Check sheet for the modelled part. Datum: model origin and axes. Units: mm. Coordinates: 2 decimals unless noted, no trailing zeros. Order: outer loops, then holes, each group sorted by start corner. A loop starts at its lowest first (then second) coordinate and runs counter-clockwise, first axis right, second up.
1. Cross-section at A-A (x = 0). Enter the section's corners in (y, z), then the cut area to 3 significant figures.
2. Thickness scan on line 1 (Z direction, x = 0, y = -5); line 2 (Z direction, x = 5.5, y = -5.25); line 3 (X direction, y = -0.5, z = -27). Record the ranges inside material, lowest first.
3. Draft check along X on faces 1 (the flat face through (0, 0, 12)), 2 (the cylindrical face through (-2.423, -3.506, 26.134)). Enter one of: released by +X, released by -X, zero draft, split by the parting line, or undercut.
4. Gauge pin test, flat ends, axial feed: pin 1 Ø1 at (x, y) = (0.5, -4.5) entering from -Z; pin 2 Ø1 at (y, z) = (-6, -38.5) entering from -X; pin 3 Ø4 at (x, y) = (-9, -1) entering from -Z; pin 4 Ø3 at (y, z) = (-6.5, -6.5) entering from +X. Record the tip position at first contact, or that the pin passes through.
5. Cross-section at C-C (y = -2). Enter the section's corners in (x, z), then the cut area to 3 significant figures.
6. Cross-section at B-B (x = 13). Enter the section's corners in (y, z), then the cut area to 3 significant figures.
```python
from build123d import *

# Parameters (mm, degrees)
F0_R         = 11.176
F1_DEPTH     = 7.112
F2_T4_ANGLE  = 116.1586222886
F2_S5_R      = 15.24
F2_T6_DEPTH  = 30
F2_S7_R      = 15.24
F2_T8_DEPTH  = 30
F2_T12_ANGLE = 116.1586222886
F2_S13_R     = 15.24
F2_T14_DEPTH = 30
F2_S15_R     = 15.24
F2_T16_DEPTH = 30
F3_R         = 5.08
F4_T4_ANGLE  = 101.759749901
F4_S5_R      = 15.24
F4_T6_DEPTH  = 23
F4_S7_R      = 15.24
F4_T8_DEPTH  = 23
F4_T12_ANGLE = 101.7597499017
F4_S13_R     = 15.24
F4_T14_DEPTH = 27
F4_S15_R     = 15.24
F4_T16_DEPTH = 27
F4_T20_ANGLE = 101.7597499014
F4_S21_R     = 15.24
F4_T22_DEPTH = 27
F4_S23_R     = 15.24
F4_T24_DEPTH = 27
F4_T28_ANGLE = 101.7597499014
F4_S29_R     = 15.24
F4_T30_DEPTH = 27
F4_S31_R     = 15.24
F4_T32_DEPTH = 27


# Not quite as in the source:
# - a fillet or chamfer that OpenCascade refuses, or shapes differently, is made with other operations: its cross-section is extruded or revolved along the edge and cut away or added


with BuildPart() as f1:
    # F0 (on Front) → F1 (new body)
    with BuildSketch(Plane.XZ):
        with BuildLine():
            ThreePointArc((10.3608125449, -11.1763662883), (13.9670394713, -6.0974919769), (15.24, 0))
            ThreePointArc((15.24, 0), (13.9670394713, 6.0974919769), (10.3608125449, 11.1763662883))
            ThreePointArc((10.3608125449, 11.1763662883), (0, 15.24), (-10.3608125449, 11.1763662883))
            ThreePointArc((-10.3608125449, 11.1763662883), (-15.24, 0), (-10.3608125449, -11.1763662883))
            ThreePointArc((-10.3608125449, -11.1763662883), (0, -15.24), (10.3608125449, -11.1763662883))
        make_face()
        Circle(F0_R, mode=Mode.SUBTRACT)
        with BuildLine():
            ThreePointArc((-10.3608125449, 11.1763662883), (0, 15.24), (10.3608125449, 11.1763662883))
            ThreePointArc((10.3608125449, 11.1763662883), (9.1357508424, 18.8221602784), (10.8748760535, 26.3676480303))
            ThreePointArc((10.8748760535, 26.3676480303), (0, 21.8044767177), (-10.8748760535, 26.3676480303))
            ThreePointArc((-10.8748760535, 26.3676480303), (-9.1357508424, 18.8221602784), (-10.3608125449, 11.1763662883))
        make_face()
        with BuildLine():
            ThreePointArc((10.8748760535, -26.3676480303), (9.1357508424, -18.8221602784), (10.3608125449, -11.1763662883))
            ThreePointArc((10.3608125449, -11.1763662883), (0, -15.24), (-10.3608125449, -11.1763662883))
            ThreePointArc((-10.3608125449, -11.1763662883), (-9.1357508424, -18.8221602784), (-10.8748760535, -26.3676480303))
            ThreePointArc((-10.8748760535, -26.3676480303), (0, -21.8044767177), (10.8748760535, -26.3676480303))
        make_face()
        with BuildLine():
            ThreePointArc((-10.8748760535, 26.3676480303), (0, 21.8044767177), (10.8748760535, 26.3676480303))
            ThreePointArc((10.8748760535, 26.3676480303), (14.1065713598, 31.2771337877), (15.24, 37.0444767177))
            ThreePointArc((15.24, 37.0444767177), (-5.76734293, 51.1510480775), (-10.8748760535, 26.3676480303))
        make_face()
        with Locations((0, 37.0444767177)):
            Circle(F0_R, mode=Mode.SUBTRACT)
        with BuildLine():
            ThreePointArc((15.24, -37.0444767177), (14.1065713598, -31.2771337877), (10.8748760535, -26.3676480303))
            ThreePointArc((10.8748760535, -26.3676480303), (0, -21.8044767177), (-10.8748760535, -26.3676480303))
            ThreePointArc((-10.8748760535, -26.3676480303), (-5.76734293, -51.1510480775), (15.24, -37.0444767177))
        make_face()
        with Locations((0, -37.0444767177)):
            Circle(F0_R, mode=Mode.SUBTRACT)
    extrude(amount=F1_DEPTH)

    # F2: fillet of radius 5.08 on 2 edges, made by hand


with BuildPart() as f2_tool2:
    # F2_s3 → F2_t4 (revolve)
    with BuildSketch(Plane(origin=(29.8644460088, 0, -17.2301380427), x_dir=(0, 1, 0), z_dir=(0.8661774261, 0, -0.4997365971))):
        with BuildLine():
            ThreePointArc((-5.08, -21.2648569422), (-1.4878975516, -22.7527544938), (0, -26.3448569422))
            Line((0, -26.3448569422), (0, -21.2648569422))
            Line((0, -21.2648569422), (-5.08, -21.2648569422))
        make_face()
    revolve(axis=Axis((29.340401561, 0, -18.1384474874), (0, 1, 0)), revolution_arc=F2_T4_ANGLE)

    # F2_s5 → F2_t6 (cut, symmetric)
    with BuildSketch(Plane.XZ.offset(2.5)):
        with Locations((0, -37.0444767177)):
            Circle(F2_S5_R)
    extrude(amount=F2_T6_DEPTH, both=True, mode=Mode.SUBTRACT)

    # F2_s7 → F2_t8 (cut, symmetric)
    with BuildSketch(Plane.XZ.offset(2.5)):
        Circle(F2_S7_R)
    extrude(amount=F2_T8_DEPTH, both=True, mode=Mode.SUBTRACT)


with BuildPart() as f1_1:
    add(f1.part)

    # F2_t1: cut F2_tool2
    add(f2_tool2.part, mode=Mode.SUBTRACT)


with BuildPart() as f2_tool10:
    # F2_s11 → F2_t12 (revolve)
    with BuildSketch(Plane(origin=(-11.8407369211, 0, 7.9442927806), x_dir=(0, 1, 0), z_dir=(-0.8304131044, 0, 0.5571481635))):
        with BuildLine():
            ThreePointArc((-5.08, 11.1931397161), (-1.4878975516, 9.7052421646), (0, 6.1131397161))
            Line((0, 6.1131397161), (0, 11.1931397161))
            Line((0, 11.1931397161), (-5.08, 11.1931397161))
        make_face()
    revolve(axis=Axis((-29.340401561, 0, -18.1384474874), (0, 1, 0)), revolution_arc=F2_T12_ANGLE)

    # F2_s13 → F2_t14 (cut, symmetric)
    with BuildSketch(Plane.XZ.offset(4.3)):
        Circle(F2_S13_R)
    extrude(amount=F2_T14_DEPTH, both=True, mode=Mode.SUBTRACT)

    # F2_s15 → F2_t16 (cut, symmetric)
    with BuildSketch(Plane.XZ.offset(4.3)):
        with Locations((0, -37.0444767177)):
            Circle(F2_S15_R)
    extrude(amount=F2_T16_DEPTH, both=True, mode=Mode.SUBTRACT)


with BuildPart() as f1_2:
    add(f1_1.part)

    # F2_t9: cut F2_tool10
    add(f2_tool10.part, mode=Mode.SUBTRACT)

    # F3#2 (call 1 of 2: OpenCascade refuses the feature's edges together)
    f3_2_edges = [f1_2.edges().sort_by_distance(p)[0] for p in [
        (-9.135751, 0, 18.82216),
    ]]
    fillet(f3_2_edges, radius=F3_R)

    # F3 (call 2 of 2)
    f3_edges = [f1_2.edges().sort_by_distance(p)[0] for p in [
        (9.135751, 0, 18.82216),
    ]]
    fillet(f3_edges, radius=F3_R)

    # F4: fillet of radius 5.08 on 4 edges, made by hand


with BuildPart() as f4_tool2:
    # F4_s3 → F4_t4 (revolve)
    with BuildSketch(Plane(origin=(27.3577839274, 0, -20.7521533482), x_dir=(0, 1, 0), z_dir=(0.7967197018, 0, -0.6043490025))):
        with BuildLine():
            ThreePointArc((-7.112, -20.9996316731), (-6.5756901303, -18.727786608), (-5.08, -16.9356316731))
            Line((-5.08, -16.9356316731), (-7.112, -16.9356316732))
            Line((-7.112, -16.9356316732), (-7.112, -20.9996316731))
        make_face()
    revolve(axis=Axis((29.340401561, -7.112, -18.1384474874), (0, 1, 0)), revolution_arc=F4_T4_ANGLE)

    # F4_s5 → F4_t6 (cut, symmetric)
    with BuildSketch(Plane.XZ.offset(4.6)):
        Circle(F4_S5_R)
    extrude(amount=F4_T6_DEPTH, both=True, mode=Mode.SUBTRACT)

    # F4_s7 → F4_t8 (cut, symmetric)
    with BuildSketch(Plane.XZ.offset(4.6)):
        with Locations((0, -37.0444767177)):
            Circle(F4_S7_R)
    extrude(amount=F4_T8_DEPTH, both=True, mode=Mode.SUBTRACT)


with BuildPart() as f1_3:
    add(f1_2.part)

    # F4_t1: cut F4_tool2
    add(f4_tool2.part, mode=Mode.SUBTRACT)


with BuildPart() as f4_tool10:
    # F4_s11 → F4_t12 (revolve)
    with BuildSketch(Plane(origin=(-7.6988506956, 0, 6.7062600285), x_dir=(0, 1, 0), z_dir=(-0.7540423315, 0, 0.6568258234))):
        with BuildLine():
            ThreePointArc((-7.112, 8.6684750316), (-6.5756901303, 10.9403200968), (-5.08, 12.7324750316))
            Line((-5.08, 12.7324750316), (-7.112, 12.7324750316))
            Line((-7.112, 12.7324750316), (-7.112, 8.6684750316))
        make_face()
    revolve(axis=Axis((-29.340401561, -7.112, -18.1384474874), (0, 1, 0)), revolution_arc=F4_T12_ANGLE)

    # F4_s13 → F4_t14 (cut, symmetric)
    with BuildSketch(Plane.XZ.offset(4.6)):
        with Locations((0, -37.0444767177)):
            Circle(F4_S13_R)
    extrude(amount=F4_T14_DEPTH, both=True, mode=Mode.SUBTRACT)

    # F4_s15 → F4_t16 (cut, symmetric)
    with BuildSketch(Plane.XZ.offset(4.6)):
        Circle(F4_S15_R)
    extrude(amount=F4_T16_DEPTH, both=True, mode=Mode.SUBTRACT)


with BuildPart() as f1_4:
    add(f1_3.part)

    # F4_t9: cut F4_tool10
    add(f4_tool10.part, mode=Mode.SUBTRACT)


with BuildPart() as f4_tool18:
    # F4_s19 → F4_t20 (revolve)
    with BuildSketch(Plane(origin=(-27.3577839275, 0, 20.7521533481), x_dir=(0, 1, 0), z_dir=(-0.7967197018, 0, 0.6043490025))):
        with BuildLine():
            ThreePointArc((-7.112, -20.9996316733), (-6.5756901303, -18.7277866081), (-5.08, -16.9356316733))
            Line((-5.08, -16.9356316733), (-7.112, -16.9356316733))
            Line((-7.112, -16.9356316733), (-7.112, -20.9996316733))
        make_face()
    revolve(axis=Axis((-29.340401561, -7.112, 18.1384474874), (0, 1, 0)), revolution_arc=F4_T20_ANGLE)

    # F4_s21 → F4_t22 (cut, symmetric)
    with BuildSketch(Plane.XZ.offset(4.6)):
        with Locations((0, 37.0444767177)):
            Circle(F4_S21_R)
    extrude(amount=F4_T22_DEPTH, both=True, mode=Mode.SUBTRACT)

    # F4_s23 → F4_t24 (cut, symmetric)
    with BuildSketch(Plane.XZ.offset(4.6)):
        Circle(F4_S23_R)
    extrude(amount=F4_T24_DEPTH, both=True, mode=Mode.SUBTRACT)


with BuildPart() as f1_5:
    add(f1_4.part)

    # F4_t17: cut F4_tool18
    add(f4_tool18.part, mode=Mode.SUBTRACT)


with BuildPart() as f4_tool26:
    # F4_s27 → F4_t28 (revolve)
    with BuildSketch(Plane(origin=(7.6988506955, 0, -6.7062600285), x_dir=(0, 1, 0), z_dir=(0.7540423315, 0, -0.6568258234))):
        with BuildLine():
            ThreePointArc((-5.08, 12.7324750317), (-6.5756901303, 10.9403200968), (-7.112, 8.6684750317))
            Line((-7.112, 8.6684750317), (-7.112, 12.7324750317))
            Line((-7.112, 12.7324750317), (-5.08, 12.7324750317))
        make_face()
    revolve(axis=Axis((29.340401561, -7.112, 18.1384474874), (0, 1, 0)), revolution_arc=F4_T28_ANGLE)

    # F4_s29 → F4_t30 (cut, symmetric)
    with BuildSketch(Plane.XZ.offset(4.6)):
        Circle(F4_S29_R)
    extrude(amount=F4_T30_DEPTH, both=True, mode=Mode.SUBTRACT)

    # F4_s31 → F4_t32 (cut, symmetric)
    with BuildSketch(Plane.XZ.offset(4.6)):
        with Locations((0, 37.0444767177)):
            Circle(F4_S31_R)
    extrude(amount=F4_T32_DEPTH, both=True, mode=Mode.SUBTRACT)


with BuildPart() as f1_6:
    add(f1_5.part)

    # F4_t25: cut F4_tool26
    add(f4_tool26.part, mode=Mode.SUBTRACT)


solid = f1_6.part
```
Data:
1. outline: (-7.11, -52.28) - (0, -52.28) - (0, -48.22) - (-7.11, -48.22) - close; (-7.11, -25.87) - (0, -25.87) - (0, -11.18) - (-7.11, -11.18) - close; (-7.11, 11.18) - (0, 11.18) - (0, 25.87) - (-7.11, 25.87) - close; (-7.11, 48.22) - (0, 48.22) - (0, 52.28) - (-7.11, 52.28) - close
1. area: 267 mm2
2. line 1: z = -52.28 to -48.22, -25.87 to -11.18, 11.18 to 25.87, 48.22 to 52.28
2. line 2: z = -51.26 to -46.77, -27.32 to -9.73, 9.73 to 27.32, 46.77 to 51.26
2. line 3: x = -11.46 to -4.9, 4.9 to 11.46
3. face 1: zero draft
3. face 2: undercut
4. pin 1: stops at z = -52.28
4. pin 2: stops at x = -15.21
4. pin 3: stops at z = -50.58
4. pin 4: stops at x = 14.4
5. outline: (-9.18, -24.88) arc R15.24 ccw (long way) to (9.18, -24.88) arc R21.26 cw to (8.88, -12.39) arc R15.24 ccw to (8.88, 12.39) arc R21.26 cw to (9.18, 24.88) arc R15.24 ccw (long way) to (-9.18, 24.88) arc R21.26 cw to (-8.88, 12.39) arc R15.24 ccw to (-8.88, -12.39) arc R21.26 cw to start; hole circle Ø22.35 at (0, -37.04); hole circle Ø22.35 at (0, 0); hole circle Ø22.35 at (0, 37.04)
5. area: 1,290 mm2
6. outline: (-7.11, -45) - (0, -45) - (0, -29.09) - (-7.11, -29.09) - close; (-7.11, -7.95) - (0, -7.95) - (0, 7.95) - (-7.11, 7.95) - close; (-7.11, 29.09) - (0, 29.09) - (0, 45) - (-7.11, 45) - close
6. area: 339 mm2
